For this review, take the finished solid that the model builds, in its own axes (mm). Face numbers are marked on the shaded views. A direction names the side the tool comes from. Coordinates: 2 decimals unless noted, no trailing zeros. Loops run counter-clockwise (first coordinate to the right, second up) from the corner with the lowest first, then second, coordinate; pieces in that order, holes last. Notation, with made-up numbers: M -39.75,29 L -26.75,29 A31 ccw -26.75,62 Z; hole C 79.25,-20.75 d9. An arc over 180 degrees is marked long. Write item = value, one per line.
from build123d import *

# Parameters (mm, degrees)
SKETCH_1_W          = 11.5
SKETCH_1_H          = 5
SKETCH_2_R          = 10.5
CUT_EXTRUDE_1_DEPTH = 4
SKETCH_3_R          = 8.5
EXTRUDE_1_DEPTH     = 10
SKETCH_4_R          = 9.5
EXTRUDE_2_DEPTH     = 5
SKETCH_5_W          = 20
SKETCH_5_H          = 20
EXTRUDE_3_DEPTH     = 1
SKETCH_6_R          = 9.5
EXTRUDE_4_DEPTH     = 9
SKETCH_7_R          = 8
EXTRUDE_5_DEPTH     = 12
FILLET_1_R          = 1


with BuildPart() as part:
    # 草图1 → 旋转1 (revolve)
    with BuildSketch(Plane(origin=(0, 0, 0), x_dir=(1, 0, 0), z_dir=(0, 1, 0))):
        with Locations((5.75, -2.5)):
            Rectangle(SKETCH_1_W, SKETCH_1_H)
    revolve(axis=Axis((0, 0, 0), (0, 0, 1)))

    # 草图2 → 切除-拉伸1 (cut)
    with BuildSketch(Plane(origin=(0, 0, 0), x_dir=(-1, 0, 0), z_dir=(0, 0, -1))):
        with Locations(Location((0, 0, 0), (0, 0, 180))):
            Circle(SKETCH_2_R)
    extrude(amount=-CUT_EXTRUDE_1_DEPTH, mode=Mode.SUBTRACT)

    # 草图3 → 凸台-拉伸1 (add)
    with BuildSketch(Plane(origin=(0, 0, 4), x_dir=(-1, 0, 0), z_dir=(0, 0, -1))):
        with Locations(Location((0, 0, 0), (0, 0, 180))):
            Circle(SKETCH_3_R)
    extrude(amount=EXTRUDE_1_DEPTH)

    # 草图4 → 凸台-拉伸2 (add)
    with BuildSketch(Plane.XY.offset(-6)):
        with Locations(Location((0, 0, 0), (0, 0, 180))):
            Circle(SKETCH_4_R)
    extrude(amount=-EXTRUDE_2_DEPTH)

    # 草图5 → 凸台-拉伸3 (add)
    with BuildSketch(Plane.XY.offset(-11)):
        Rectangle(SKETCH_5_W, SKETCH_5_H)
    extrude(amount=-EXTRUDE_3_DEPTH)

    # 草图6 → 凸台-拉伸4 (add)
    with BuildSketch(Plane(origin=(0, 0, -12), x_dir=(-1, 0, 0), z_dir=(0, 0, -1))):
        Circle(SKETCH_6_R)
    extrude(amount=EXTRUDE_4_DEPTH)

    # 草图7 → 凸台-拉伸5 (add)
    with BuildSketch(Plane(origin=(0, 0, -21), x_dir=(-1, 0, 0), z_dir=(0, 0, -1))):
        Circle(SKETCH_7_R)
    extrude(amount=EXTRUDE_5_DEPTH)

    # 圆角1
    fillet_1_edges = [part.edges().sort_by_distance(p)[0] for p in [
        (-11.5, 0, 5),
    ]]
    fillet(fillet_1_edges, radius=FILLET_1_R)


solid = part.part
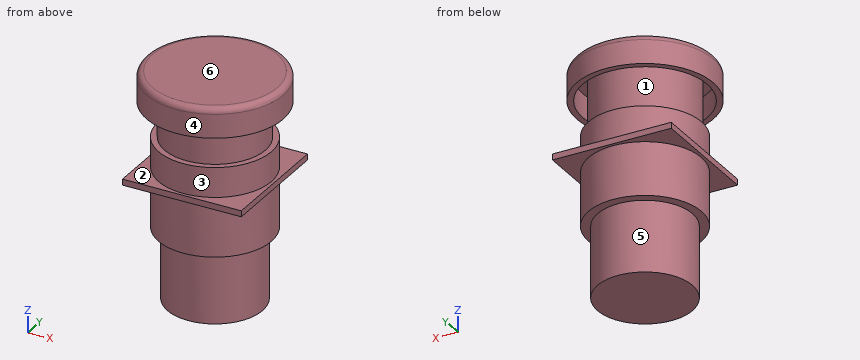
Q1. For pin 1 Ø2 at (x, z) = (-6, -0.5) entering from +Y; pin 2 Ø3 at (y, z) = (-7, -7.5) entering from -X; pin 3 Ø1.1 at (y, z) = (-4, -11.5) entering from -X, all flat-tipped, find the tip position at first contact; note any pin that passes through.
Solved:
pin_1 = 10.29
pin_2 = -7.75
pin_3 = -10
Q2. For line 1 along Y through (x, z) = (0, 2.4); line 2 along Z through (x, y) = (-3.75, -8.25); line 3 along Z through (x, y) = (-7, 8), list the stretches that pass through material, from the lowest coordinate up.
Solved:
line_1 = -11.5 to -10.5, -8.5 to 8.5, 10.5 to 11.5
line_2 = -21 to -6, 4 to 5
line_3 = -12 to -11, 0 to 4.99
Q3. Machinability: for the marked faces 4, 5 and 6, which of the approach directions +Z, -Z, +X, -X, +Y, -Y give a long, thin tool a straight path to every point of the face, cutting with its end or side? Answer none if there is none.
Solved:
face_4 = +Z
face_5 = -Z
face_6 = +Z, +X, -X, +Y, -Y
Q4. Add section C-C (z = -7). Write out the cut boundary in (x, y), and give its area (3 significant figures).
Solved:
outline = C 0,0 d19
area = 284 mm²
Q5. Draft analysis for pull direction X (two halves, no side actions). For the marked faces 1, 2 and 3, state which applies: +X half, -X half, draft (parallel to the pull), parting line (faces both ways), or undercut.
Solved:
face_1 = undercut
face_2 = draft
face_3 = parting line
